from build123d import *

# Parameters (mm, degrees)
SKETCH_1_R        = 6
SKETCH_1_R_2      = 3
EXTRUDE_1_DEPTH   = 9
EXTRUDE_1_2_DEPTH = 9
EXTRUDE_1_3_DEPTH = 9
EXTRUDE_1_4_DEPTH = 9
SKETCH_2_W        = 140
SKETCH_2_H        = 90
SKETCH_2_R        = 2.5
EXTRUDE_2_DEPTH   = 3
FILLET_1_R        = 3


with BuildPart() as part:
    # Sketch 1 → Extrude 1 (new body)
    with BuildSketch(Plane(origin=(0, 0, 0), x_dir=(1, 0, 0), z_dir=(0, 1, 0))):
        with Locations(Location((-34.925000029, 23.728220461, 0), (0, 0, 270))):
            Circle(SKETCH_1_R)
        with Locations(Location((-34.925000029, 23.728220461, 0), (0, 0, 270))):
            Circle(SKETCH_1_R_2, mode=Mode.SUBTRACT)
    extrude(amount=-EXTRUDE_1_DEPTH)



with BuildPart() as body_2:
    # Sketch 1 → Extrude 1 2 (new body)
    with BuildSketch(Plane(origin=(0, 0, 0), x_dir=(1, 0, 0), z_dir=(0, 1, 0))):
        with Locations(Location((40.004999984, 23.728220453, 0), (0, 0, 270))):
            Circle(SKETCH_1_R)
        with Locations(Location((40.004999984, 23.728220453, 0), (0, 0, 270))):
            Circle(SKETCH_1_R_2, mode=Mode.SUBTRACT)
    extrude(amount=-EXTRUDE_1_2_DEPTH)


with BuildPart() as body_3:
    # Sketch 1 → Extrude 1 3 (new body)
    with BuildSketch(Plane(origin=(0, 0, 0), x_dir=(1, 0, 0), z_dir=(0, 1, 0))):
        with Locations(Location((41.275000034, -24.53177948, 0), (0, 0, 270))):
            Circle(SKETCH_1_R)
        with Locations(Location((41.275000034, -24.53177948, 0), (0, 0, 270))):
            Circle(SKETCH_1_R_2, mode=Mode.SUBTRACT)
    extrude(amount=-EXTRUDE_1_3_DEPTH)


with BuildPart() as body_4:
    # Sketch 1 → Extrude 1 4 (new body)
    with BuildSketch(Plane(origin=(0, 0, 0), x_dir=(1, 0, 0), z_dir=(0, 1, 0))):
        with Locations(Location((-41.275000034, -24.531779532, 0), (0, 0, 270))):
            Circle(SKETCH_1_R)
        with Locations(Location((-41.275000034, -24.531779532, 0), (0, 0, 270))):
            Circle(SKETCH_1_R_2, mode=Mode.SUBTRACT)
    extrude(amount=-EXTRUDE_1_4_DEPTH)


with BuildPart() as part_1:
    add(part.part)

    add(body_2.part)  # Extrude 2 merges body 2

    add(body_3.part)  # Extrude 2 merges body 3

    add(body_4.part)  # Extrude 2 merges body 4
    # Sketch 2 → Extrude 2 (add)
    with BuildSketch(Plane(origin=(0, 0, 0), x_dir=(1, 0, 0), z_dir=(0, 1, 0))):
        with Locations((-0.274084252, -0.781638626)):
            Rectangle(SKETCH_2_W, SKETCH_2_H)
        with Locations(Location((-64.274084252, 38.218361374, 0), (0, 0, 270))):
            Circle(SKETCH_2_R, mode=Mode.SUBTRACT)
        with Locations(Location((63.725915748, 38.218361374, 0), (0, 0, 90))):
            Circle(SKETCH_2_R, mode=Mode.SUBTRACT)
        with Locations(Location((63.725915748, -39.781638626, 0), (0, 0, 270))):
            Circle(SKETCH_2_R, mode=Mode.SUBTRACT)
        with Locations(Location((-64.274084252, -39.781638626, 0), (0, 0, 90))):
            Circle(SKETCH_2_R, mode=Mode.SUBTRACT)
    extrude(amount=-EXTRUDE_2_DEPTH)

    # Fillet 1
    fillet_1_edges = [part_1.edges().sort_by_distance(p)[0] for p in [
        (69.725915748, -1.5, -44.218361374),
        (69.725915748, -1.5, 45.781638626),
        (-70.274084252, -1.5, 45.781638626),
        (-70.274084252, -1.5, -44.218361374),
    ]]
    fillet(fillet_1_edges, radius=FILLET_1_R)


solid = part_1.part
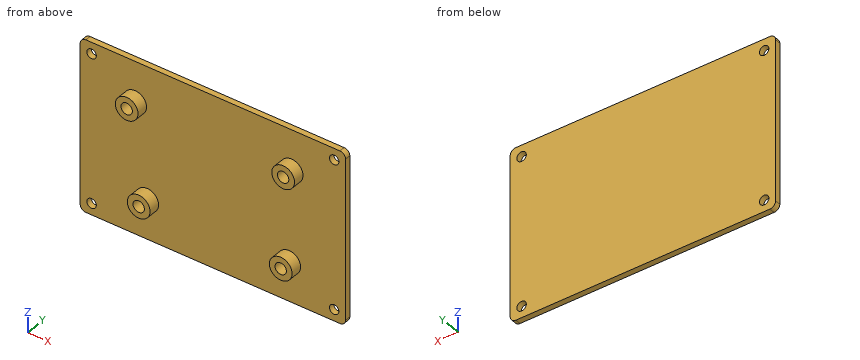
Read the model definition and answer for the solid it produces. Units are mm, in the model's axes. Round coordinates to 2 decimals unless told otherwise and drop trailing zeros. Loops run counter-clockwise (first coordinate to the right, second up) from the corner with the lowest first, then second, coordinate; pieces in that order, holes last.
Q1. Section C-C on x = 57 is taken. Write down the section's boundary in (y, z), and give its area (3 significant figures).
Q2. Consider probe 1 along X at (y, z) = (-5, 24.5); probe 2 along X at (y, z) = (-4.25, -21); probe 3 along Z at (x, y) = (42.5, -7). Determine where each line is inside the solid, lowest interval first.
Q3. Each of these flat-tipped pins is pushed along its axis until it touches: pin 1 (2 mm diameter, centred on x = 38.5, y = -6, fed in from -Z); pin 2 (4 mm diameter, centred on x = -64.27, z = 39.78, fed in from -Y); pin 3 (2 mm diameter, centred on x = -32.5, z = 26, fed in from +Y); pin 4 (3 mm diameter, centred on x = 39.5, z = -25, fed in from -Y). Where does it stop, or does it pass through?
Q4. Section B-B on z = 8 is taken. Write down the section's boundary in (x, y).
Q5. Section A-A on y = -5 is taken. Write down the section's boundary in (x, z) (3 decimals).
Output:
1. outline: (-3, -44.22) - (0, -44.22) - (0, 45.78) - (-3, 45.78) - close
1. area: 270 mm2
2. probe 1: x = -47.27 to -44.27, -38.28 to -35.28, 35.28 to 38.28, 44.27 to 47.27
2. probe 2: x = -40.27 to -36.17, -33.68 to -29.58, 34.66 to 38.76, 41.25 to 45.35
2. probe 3: z = -29.18 to -25.39, -22.06 to -18.27, 18.66 to 21.79, 27.27 to 30.41
3. pin 1: stops at z = -29.71
3. pin 2: passes through
3. pin 3: stops at y = 0
3. pin 4: stops at y = -3
4. outline: (-70.27, -3) - (69.73, -3) - (69.73, 0) - (-70.27, 0) - close
5. outline: circle Ø12 at (-41.275, 24.532); circle Ø12 at (-34.925, -23.728); circle Ø12 at (40.005, -23.728); circle Ø12 at (41.275, 24.532); hole circle Ø6 at (-41.275, 24.532); hole circle Ø6 at (-34.925, -23.728); hole circle Ø6 at (40.005, -23.728); hole circle Ø6 at (41.275, 24.532)
